from build123d import *

# Parameters (mm, degrees)
BOSS_EXTRU_1_DEPTH      = 120
CONG_1_R                = 3
ESQUISSE3_W             = 57.5
ESQUISSE3_H             = 57.5
ENL_V_MAT_EXTRU_1_DEPTH = 17.5
ESQUISSE4_W             = 120
ESQUISSE4_H             = 120
ESQUISSE4_W_2           = 115
ESQUISSE4_H_2           = 115
BOSS_EXTRU_2_DEPTH      = 30
CONG_2_R                = 3


with BuildPart() as part:
    # Esquisse2 → Boss.-Extru.1 (new body)
    with BuildSketch(Plane(origin=(0, 0, 0), x_dir=(0, 0, -1), z_dir=(1, 0, 0))):
        Polygon((0, 20), (0, 0), (118.743991381, 0), (120, 0), (120, 20), align=None)
    extrude(amount=BOSS_EXTRU_1_DEPTH)

    # Congé1
    cong_1_edges = [part.edges().sort_by_distance(p)[0] for p in [
        (120, 10, 0),
        (0, 10, 0),
    ]]
    fillet(cong_1_edges, radius=CONG_1_R)

    # Esquisse3 → Enlèv. mat.-Extru.1 (cut)
    with BuildSketch(Plane(origin=(0, 20, 0), x_dir=(1, 0, 0), z_dir=(0, 1, 0))):
        with Locations((31.25, 88.75)):
            Rectangle(ESQUISSE3_W, ESQUISSE3_H)
        with Locations((88.75, 88.75)):
            Rectangle(ESQUISSE3_W, ESQUISSE3_H)
        with Locations((31.25, 31.25)):
            Rectangle(ESQUISSE3_W, ESQUISSE3_H)
        with Locations((88.75, 31.25)):
            Rectangle(ESQUISSE3_W, ESQUISSE3_H)
    extrude(amount=-ENL_V_MAT_EXTRU_1_DEPTH, mode=Mode.SUBTRACT)

    # Esquisse4 → Boss.-Extru.2 (add)
    with BuildSketch(Plane(origin=(0, 20, 0), x_dir=(1, 0, 0), z_dir=(0, 1, 0))):
        with Locations((60, 60)):
            Rectangle(ESQUISSE4_W, ESQUISSE4_H)
        with Locations((60, 60)):
            Rectangle(ESQUISSE4_W_2, ESQUISSE4_H_2, mode=Mode.SUBTRACT)
    extrude(amount=BOSS_EXTRU_2_DEPTH)

    # Congé2
    cong_2_edges = [part.edges().sort_by_distance(p)[0] for p in [
        (120, 35, 0),
        (0, 35, 0),
    ]]
    fillet(cong_2_edges, radius=CONG_2_R)


solid = part.part
Can you work these out from the model? Positions are in its coordinate system, mm. A direction names the side the tool comes from. Coordinates: 2 decimals unless noted, no trailing zeros. Loops run counter-clockwise (first coordinate to the right, second up) from the corner with the lowest first, then second, coordinate; pieces in that order, holes last. Notation, with made-up numbers: M 78,-7 L 84,-7 A17 ccw 84,23 Z; hole C -31,18.5 d5. An arc over 180 degrees is marked long. Return JSON: item names as keys, results as strings. Group by question number.
Item 1: I'm going to push a flat-ended pin straight in: pin 1 Ø3 at (x, z) = (97, -89.5) entering from +Y. Where does the tip first touch, or does it pass through?
Item 2: Imagine slicing it at C-C (z = -80.5). Please give me the cut outline in (x, y).
Item 3: Thinking about a two-plate mould opening in Z: for faces 3 (the cylindrical face through (119.14, 35.21, -0.9)), 4 (the flat face through (59, 26, -2.5)), 5 (the flat face through (59, 0, -59)), which applies, released by +Z, released by -Z, zero draft, split by the parting line, or undercut?
Item 4: Imagine slicing it at A-A (y = 46). Please give me the cut outline in (x, z).
Item 5: On a 3-axis mill with a long thin cutter (end or side, diameter ignored), from which of +Z, -Z, +X, -X, +Y, -Y can I reach the whole of each face in a straight line? I mean faces 1 (the flat face through (0, 25, -61)), 2 (the flat face through (59, 26, -117.5)). Say none if no direction works.
Item 6: If I drill on L1, parallel to X at y = 34.5, z = -102; L2, parallel to Z at x = 50, y = 22; L3, parallel to Y at x = 81, z = -31, over which ranges is the centre line in solid material (lowest first)? Write a range as from..to.
Item 7: Imagine slicing it at B-B (x = 112). Please give me the cut outline in (y, z).
Verdict:
{
 "1": {"pin 1": "stops at y = 2.5"},
 "2": {"outline": "M 0,0 L 120,0 L 120,50 L 117.5,50 L 117.5,2.5 L 2.5,2.5 L 2.5,50 L 0,50 Z"},
 "3": {"face 3": "released by +Z", "face 4": "undercut", "face 5": "zero draft"},
 "4": {"outline": "M 0,-120 L 120,-120 L 120,-3 A3 ccw 117,0 L 3,0 A3 ccw 0,-3 Z; hole M 2.5,-117.5 L 117.5,-117.5 L 117.5,-2.5 L 2.5,-2.5 Z"},
 "5": {"face 1": "+Z, -Z, -X, +Y, -Y", "face 2": "+Y"},
 "6": {"L1": "x = 0..2.5, 117.5..120", "L2": "z = -120..-117.5, -2.5..0", "L3": "y = 0..2.5"},
 "7": {"outline": "M 0,-120 L 50,-120 L 50,-117.5 L 2.5,-117.5 L 2.5,-2.5 L 50,-2.5 L 50,0 L 0,0 Z"}
}
